```python
from build123d import *

# Parameters (mm, degrees)
SKETCH_1_W          = 8
SKETCH_1_H          = 8
SKETCH_1_R          = 2.1
EXTRUDE_1_DEPTH     = 1
EXTRUDE_START       = 1
SKETCH_1_6_W        = 2
SKETCH_1_6_H        = 8
EXTRUDE_2_DEPTH     = 15
EXTRUDE_2_2_DEPTH   = 15
SKETCH_2_W          = 0.9
SKETCH_2_H          = 0.6
SKETCH_2_W_2        = 6.2
SKETCH_2_H_2        = 6.8
EXTRUDE_3_DEPTH     = 4.5
CUT_EXTRUDE_1_REACH = 19.205
SKETCH_3_W          = 1.6
SKETCH_3_H          = 2
SKETCH_4_R          = 0.7
CUT_EXTRUDE_2_DEPTH = 19.867962264
SKETCH_4_3_R        = 1.1
CUT_EXTRUDE_3_DEPTH = 1
CUT_EXTRUDE_START   = -11
SKETCH_4_4_R        = 1.1
CUT_EXTRUDE_4_DEPTH = 1


with BuildPart() as part:
    # Sketch 1 → Extrude 1 (new body)
    with BuildSketch(Plane(origin=(0, 0, 0), x_dir=(1, 0, 0), z_dir=(0, 1, 0))):
        Rectangle(SKETCH_1_W, SKETCH_1_H)
        with Locations(Location((0, 0, 0), (0, 0, 270))):
            Circle(SKETCH_1_R, mode=Mode.SUBTRACT)
    extrude(amount=EXTRUDE_1_DEPTH)



with BuildPart() as body_2:
    # Sketch 1_6 → Extrude 2 (new body)
    with BuildSketch(Plane(origin=(0, 0, 0), x_dir=(1, 0, 0), z_dir=(0, 1, 0)).offset(EXTRUDE_START)):
        with Locations((-5, 0)):
            Rectangle(SKETCH_1_6_W, SKETCH_1_6_H)
    extrude(amount=-EXTRUDE_2_DEPTH)


with BuildPart() as body_3:
    # Sketch 1_6 → Extrude 2 2 (new body)
    with BuildSketch(Plane(origin=(0, 0, 0), x_dir=(1, 0, 0), z_dir=(0, 1, 0)).offset(EXTRUDE_START)):
        with Locations((5, 0)):
            Rectangle(SKETCH_1_6_W, SKETCH_1_6_H)
    extrude(amount=-EXTRUDE_2_2_DEPTH)


with BuildPart() as part_1:
    add(part.part)

    add(body_2.part)  # Extrude 3 merges body 2

    add(body_3.part)  # Extrude 3 merges body 3
    # Sketch 2 → Extrude 3 (add)
    with BuildSketch(Plane.XZ):
        with Locations((-3.55, 3.7)):
            Rectangle(SKETCH_2_W, SKETCH_2_H)
        with Locations((0, 3.7)):
            Rectangle(SKETCH_2_W_2, SKETCH_2_H)
        with Locations((3.55, 3.7)):
            Rectangle(SKETCH_2_W, SKETCH_2_H)
        with Locations((3.55, 0)):
            Rectangle(SKETCH_2_W, SKETCH_2_H_2)
        with Locations((3.55, -3.7)):
            Rectangle(SKETCH_2_W, SKETCH_2_H)
        with Locations((0, -3.7)):
            Rectangle(SKETCH_2_W_2, SKETCH_2_H)
        with Locations((-3.55, -3.7)):
            Rectangle(SKETCH_2_W, SKETCH_2_H)
        with Locations((-3.55, 0)):
            Rectangle(SKETCH_2_W, SKETCH_2_H_2)
    extrude(amount=EXTRUDE_3_DEPTH)

    # Sketch 3 → Cut-Extrude 1 (cut, up to next)
    with BuildSketch(Plane(origin=(0, 0, -4), x_dir=(-1, 0, 0), z_dir=(0, 0, -1)), mode=Mode.PRIVATE) as cut_extrude_1_sk1:
        with Locations((-2.2, -3.5)):
            Rectangle(SKETCH_3_W, SKETCH_3_H)
    cut_extrude_1_tool1 = extrude(cut_extrude_1_sk1.sketch, amount=-CUT_EXTRUDE_1_REACH, mode=Mode.PRIVATE) & part_1.part
    # Sketch 3 → Cut-Extrude 1 (cut, up to next)
    with BuildSketch(Plane(origin=(0, 0, -4), x_dir=(-1, 0, 0), z_dir=(0, 0, -1)), mode=Mode.PRIVATE) as cut_extrude_1_sk2:
        with Locations((2.2, -3.5)):
            Rectangle(SKETCH_3_W, SKETCH_3_H)
    cut_extrude_1_tool2 = extrude(cut_extrude_1_sk2.sketch, amount=-CUT_EXTRUDE_1_REACH, mode=Mode.PRIVATE) & part_1.part
    add(cut_extrude_1_tool1.solids().sort_by_distance((2.2, -3.5, -4))[0], mode=Mode.SUBTRACT)
    add(cut_extrude_1_tool2.solids().sort_by_distance((-2.2, -3.5, -4))[0], mode=Mode.SUBTRACT)

    # Sketch 4 → Cut-Extrude 2 (cut, through all)
    with BuildSketch(Plane(origin=(6, 0, 0), x_dir=(0, 0, -1), z_dir=(1, 0, 0))):
        with Locations((-2, -8)):
            Circle(SKETCH_4_R)
        with Locations((2, -11)):
            Circle(SKETCH_4_R)
    extrude(amount=-CUT_EXTRUDE_2_DEPTH, mode=Mode.SUBTRACT)

    # Sketch 4_3 → Cut-Extrude 3 (cut)
    with BuildSketch(Plane(origin=(6, 0, 0), x_dir=(0, 0, -1), z_dir=(1, 0, 0))):
        with Locations((-2, -8)):
            Circle(SKETCH_4_3_R)
        with Locations((2, -11)):
            Circle(SKETCH_4_3_R)
    extrude(amount=-CUT_EXTRUDE_3_DEPTH, mode=Mode.SUBTRACT)

    # Sketch 4_4 → Cut-Extrude 4 (cut)
    with BuildSketch(Plane(origin=(6, 0, 0), x_dir=(0, 0, -1), z_dir=(1, 0, 0)).offset(CUT_EXTRUDE_START)):
        with Locations((-2, -8)):
            Circle(SKETCH_4_4_R)
        with Locations((2, -11)):
            Circle(SKETCH_4_4_R)
    extrude(amount=-CUT_EXTRUDE_4_DEPTH, mode=Mode.SUBTRACT)


solid = part_1.part
```
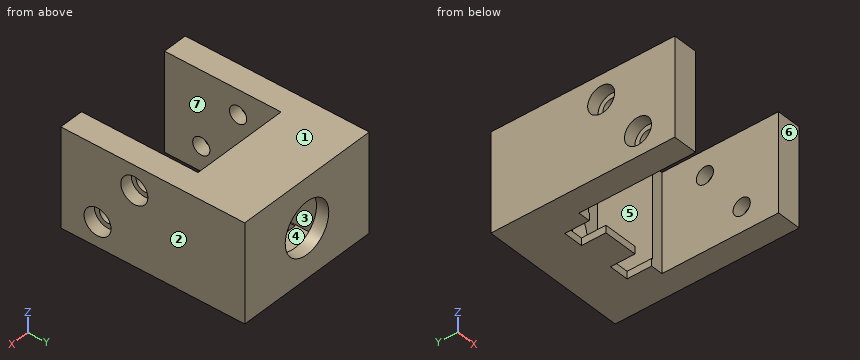
Can you work these out from the model? Positions are in its coordinate system, mm. Face numbers are marked on the shaded views. A direction names the side the tool comes from. Coordinates: 2 decimals unless noted, no trailing zeros. Loops run counter-clockwise (first coordinate to the right, second up) from the corner with the lowest first, then second, coordinate; pieces in that order, holes last. Notation, with made-up numbers: (10, -22) - (58, -22) arc R26 ccw to (58, 4) - close; hole circle Ø3 at (-27.75, 75.5). An arc over 180 degrees is marked (long way). Use a Markdown table: item, result.
Item 1: For the marked faces 5, 6 and 7, which set-ups out of +Z, -Z, +X, -X, +Y, -Y let a thin tool reach every point of the face, with its end or its side?
Numbers:
| item | result |
|---|---|
| face 5 | -Y |
| face 6 | +Z, -Z, +X, -X, -Y |
| face 7 | +Z, -Z, -Y |
Item 2: Will these pins go through, and if not, where does the flat tip stop? pin 1 (2.5 mm diameter, centred on y = -8, z = 2, fed in from +X); pin 2 (0.7 mm diameter, centred on y = -7.5, z = 2, fed in from -X); pin 3 (0.5 mm diameter, centred on x = -2, z = -3.5, fed in from -Y).
Numbers:
| item | result |
|---|---|
| pin 1 | stops at x = 6 |
| pin 2 | stops at x = -5 |
| pin 3 | stops at y = -2.5 |
Item 3: If I drill on probe 1 along X at (y, z) = (-10.25, 1.5); probe 2 along Y at (x, z) = (-5.75, 2); probe 3 along X at (y, z) = (-3, 0.25), over which ranges is the centre line in solid material (lowest first)? Write a range as from..to.
Numbers:
| item | result |
|---|---|
| probe 1 | x = -6..-4, 4..6 |
| probe 2 | y = -14..-9.1, -6.9..1 |
| probe 3 | x = -6..-3.1, 3.1..6 |
Item 4: I want a section at D-D on z = -1.75. Give the number of separate pieces and of enclosed holes in the cut face, and give its area (3 significant figures).
Numbers:
| item | result |
|---|---|
| separate pieces | 4 |
| enclosed holes | 0 |
| area | 66.9 mm2 |
Item 5: We'd pull the mould along X, two halves only. Please class the marked faces 1, 2, 3 and 4: released by +X, released by -X, zero draft, split by the parting line, or undercut.
Numbers:
| item | result |
|---|---|
| face 1 | zero draft |
| face 2 | released by +X |
| face 3 | undercut |
| face 4 | undercut |
Item 6: I want a section at B-B on z = 0. Please give me the cut outline in (x, y), and give its area (3 significant figures).
Numbers:
| item | result |
|---|---|
| outline | (-6, -14) - (-4, -14) - (-4, -4.5) - (-3.1, -4.5) - (-3.1, 0) - (-2.1, 0) - (-2.1, 1) - (-6, 1) - close; (2.1, 0) - (3.1, 0) - (3.1, -4.5) - (4, -4.5) - (4, -14) - (6, -14) - (6, 1) - (2.1, 1) - close |
| area | 71.9 mm2 |
Item 7: I want a section at A-A on y = -5. Please give me the cut outline in (x, z), and give its area (3 significant figures).
Numbers:
| item | result |
|---|---|
| outline | (-6, -4) - (-4, -4) - (-4, 4) - (-6, 4) - close; (4, -4) - (6, -4) - (6, 4) - (4, 4) - close |
| area | 32.0 mm2 |
Item 8: I want a section at C-C on y = -0.5. Please give me the cut outline in (x, z).
Numbers:
| item | result |
|---|---|
| outline | (-6, -4) - (6, -4) - (6, 4) - (-6, 4) - close; hole (-3.1, -3.4) - (3.1, -3.4) - (3.1, 3.4) - (-3.1, 3.4) - close |
